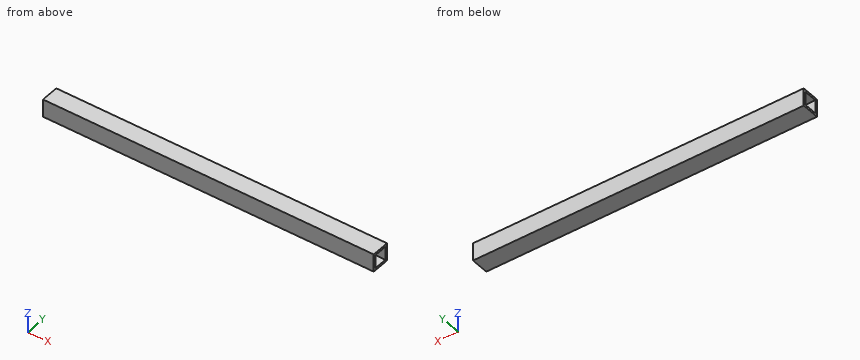
Autodesk Inventor part; units mm, degrees
ref_plane "Work Plane1" through (121.4904, -591.0492, 62.9788) normal (-1, 0, 0) x (0, -0.0011, 1)
ref_plane "Work Plane2" through (594.413, -591.0492, 62.9788) normal (1, 0, 0) x (0, 1, 0.0011)
ref_plane "Work Plane3" through (121.4904, -685.829, -0.8415) normal (-1, 0, 0) x (0, 0, 1)
sketch "Sketch1" plane through (0, 0, 0) normal (1, 0, 0) x (0, 1, 0)
  line L0 (0, 0) -> (25.4, 0)
  line L1 (25.4, 0) -> (25.4, -25.4)
  line L2 (0, 0) -> (0, -25.4)
  line L3 (0, -25.4) -> (25.4, -25.4)
  line L4 (22.225, -22.225) -> (22.225, -3.175)
  line L5 (22.225, -3.175) -> (3.175, -3.175)
  line L6 (3.175, -3.175) -> (3.175, -22.225)
  line L7 (3.175, -22.225) -> (22.225, -22.225)
  dimension "d1" = 25.4
  dimension "d5" = 25.4
  dimension "d7" = 25.4
  dimension "d8" = 3.175
ref_plane "Work Plane1" through (121.4904, -591.0492, 62.9788) normal (-1, 0, 0) x (0, -0.0011, 1)
ref_plane "Work Plane2" through (594.413, -591.0492, 62.9788) normal (1, 0, 0) x (0, 1, 0.0011)
ref_plane "Work Plane3" through (121.4904, -685.829, -0.8415) normal (-1, 0, 0) x (0, 0, 1)
ref_plane "Work Plane4" through (572.188, -685.8218, 2.3335) normal (1, 0, 0) x (0, 1, 0)
ref_plane "Work Plane5" through (571.4614, -9.58, -1.5962) normal (1, 0, 0) x (0, 1, 0)
ref_plane "Work Plane6" through (98.5388, -9.58, -1.5962) normal (-1, 0, 0) x (0, 0, 1)
extrude "Extrusion1" add sketch "Sketch1" against normal up to surface (472.9226 mm away) from surface at 571.4614 contours L0 L1 L3 L2 | L7 L6 L5 L4
ref_plane "Work Plane7" through (98.5388, -9.554, -0.8415) normal (-1, 0, 0) x (0, 0, 1)
ref_plane "Work Plane8" through (571.4614, -9.554, -0.8415) normal (1, 0, 0) x (0, 1, 0)
extrude "Extrusion2" cut sketch "Sketch1" along normal up to surface (472.9226 mm away) from surface at 98.5388 contours L7 L6 L5 L4
properties part number "15102898-16-P-0219"
Could you check a few things on this model? Use its own coordinates, in mm. Coordinates: 2 decimals unless noted, no trailing zeros. Loops run counter-clockwise (first coordinate to the right, second up) from the corner with the lowest first, then second, coordinate; pieces in that order, holes last.
1) Imagine slicing it at B-B (x = 537.5). List the corners of the cut face in (y, z) for me (3 decimals), and give its area (3 significant figures).
Reported:
outline: (0, -25.4) - (25.4, -25.4) - (25.4, 0) - (0, 0) - close; hole (3.175, -22.225) - (22.225, -22.225) - (22.225, -3.175) - (3.175, -3.175) - close
area: 282 mm2
2) Imagine slicing it at A-A (y = 16.5). List the corners of the cut face in (x, z) for me (3 decimals), and give its area (3 significant figures).
Reported:
outline: (98.539, -25.4) - (571.461, -25.4) - (571.461, -22.225) - (98.539, -22.225) - close; (98.539, -3.175) - (571.461, -3.175) - (571.461, 0) - (98.539, 0) - close
area: 3,000 mm2
3) Imagine slicing it at C-C (z = -12). List the corners of the cut face in (x, y) for me (3 decimals), and give its area (3 significant figures).
Reported:
outline: (98.539, 0) - (571.461, 0) - (571.461, 3.175) - (98.539, 3.175) - close; (98.539, 22.225) - (571.461, 22.225) - (571.461, 25.4) - (98.539, 25.4) - close
area: 3,000 mm2
4) Please list where these lines run through material, in increasing order: line 1 along Z through (x, y) = (272, 15.75) (3 decimals); line 2 along Y through (x, z) = (241, -8.75) (3 decimals).
Reported:
line 1: z = -25.4 to -22.225, -3.175 to 0
line 2: y = 0 to 3.175, 22.225 to 25.4
